The listing builds one solid part. Answer for the finished solid, in the listing's coordinates (mm). A direction names the side the tool comes from. Coordinates: 2 decimals unless noted, no trailing zeros. Order: outer loops, then holes, each group sorted by start corner. A loop starts at its lowest first (then second) coordinate and runs counter-clockwise, first axis right, second up. Notation, with made-up numbers: (71, 70.5) -> (102, 70.5) arc R15 ccw to (102, 76.5) -> close; hole circle Ø6 at (11.5, -6.75). An arc over 180 degrees is marked (long way). Answer in a Markdown table with one row per item.
```python
from build123d import *

# Parameters (mm, degrees)
SKETCH_1_W                = 5
SKETCH_1_H                = 10
EXTRUDE_1_DEPTH           = 4
CUT_EXTRUDE_1_DEPTH       = 9.124038405
CUT_EXTRUDE_1_DEPTH_BACK  = 9.124038405
CUT_EXTRUDE_2_DEPTH       = 9.124038405
CUT_EXTRUDE_2_DEPTH_BACK  = 9.124038405
SKETCH_6_W                = 4
SKETCH_6_H                = 3
CUT_EXTRUDE_3_DEPTH       = 2.5
SKETCH_7_W                = 4
SKETCH_7_H                = 3
CUT_EXTRUDE_4_DEPTH       = 2.5
CUT_EXTRUDE_5_DEPTH       = 9.124038405
CUT_EXTRUDE_5_DEPTH_BACK  = 9.124038405
CUT_EXTRUDE_10_DEPTH      = 9.124038405
CUT_EXTRUDE_10_DEPTH_BACK = 5
SKETCH_11_R               = 0.25
CUT_EXTRUDE_11_DEPTH      = 5
SKETCH_12_R               = 0.25
CUT_EXTRUDE_12_DEPTH      = 5
EXTRUDE_3_DEPTH           = 5
SCALE_1_SCALE             = 2.454545455


with BuildPart() as part:
    # Sketch 1 → Extrude 1 (new body)
    with BuildSketch(Plane.XY):
        Rectangle(SKETCH_1_W, SKETCH_1_H)
    extrude(amount=EXTRUDE_1_DEPTH)

    # Sketch 2 → Cut-Extrude 1 (cut, two sides: drawn at the far end of the back side and taken through both)
    with BuildSketch(Plane(origin=(2.5, 0, 0), x_dir=(0, 0, -1), z_dir=(1, 0, 0)).offset(-CUT_EXTRUDE_1_DEPTH_BACK)):
        Polygon((-31.620459958, -9.310229979), (-4, 4.5), (-3, 5), (24.620459958, 18.810229979), (-3, 74.051149895), (-59.240919916, 45.930689937), align=None)
    extrude(amount=CUT_EXTRUDE_1_DEPTH + CUT_EXTRUDE_1_DEPTH_BACK, mode=Mode.SUBTRACT)

    # Sketch 3 → Cut-Extrude 2 (cut, two sides: drawn at the far end of the back side and taken through both)
    with BuildSketch(Plane(origin=(2.5, 0, 0), x_dir=(0, 0, -1), z_dir=(1, 0, 0)).offset(-CUT_EXTRUDE_2_DEPTH_BACK)):
        Polygon((-3, 35.880613018), (-3, 5), (-3, -1), (0, -1), (30.880613018, -1), (76.363050598, 40.782734631), (42.48243758, 77.663347649), align=None)
    extrude(amount=CUT_EXTRUDE_2_DEPTH + CUT_EXTRUDE_2_DEPTH_BACK, mode=Mode.SUBTRACT)

    # Sketch 6 → Cut-Extrude 3 (cut)
    with BuildSketch(Plane(origin=(0, -1, 0), x_dir=(1, 0, 0), z_dir=(0, 1, 0))):
        with Locations((0, -1.5)):
            Rectangle(SKETCH_6_W, SKETCH_6_H)
    extrude(amount=-CUT_EXTRUDE_3_DEPTH, mode=Mode.SUBTRACT)

    # Sketch 7 → Cut-Extrude 4 (cut)
    with BuildSketch(Plane(origin=(0, 0, 3), x_dir=(-1, 0, 0), z_dir=(0, 0, -1))):
        with Locations((0, 3.5)):
            Rectangle(SKETCH_7_W, SKETCH_7_H)
    extrude(amount=-CUT_EXTRUDE_4_DEPTH, mode=Mode.SUBTRACT)

    # Sketch 8 → Cut-Extrude 5 (cut, two sides: drawn at the far end of the back side and taken through both)
    with BuildSketch(Plane(origin=(2.5, 0, 0), x_dir=(0, 0, -1), z_dir=(1, 0, 0)).offset(-CUT_EXTRUDE_5_DEPTH_BACK)):
        Polygon((-25.835890872, 17.835890872), (-4, -4), (-3, -5), (18.835890872, -26.835890872), (-24.835890872, -70.507672616), (-69.507672616, -25.835890872), align=None)
    extrude(amount=CUT_EXTRUDE_5_DEPTH + CUT_EXTRUDE_5_DEPTH_BACK, mode=Mode.SUBTRACT)

    # Sketch 9 → Cut-Extrude 10 (cut, two sides: drawn at the far end of the back side and taken through both)
    with BuildSketch(Plane(origin=(2.5, 0, 0), x_dir=(0, 0, -1), z_dir=(1, 0, 0)).offset(-CUT_EXTRUDE_10_DEPTH_BACK)):
        Polygon((-23.148447549, -26.648447549), (-1.5, -5), (0, -3.5), (21.648447549, 18.148447549), (64.945342647, -25.148447549), (20.148447549, -69.945342647), align=None)
    extrude(amount=CUT_EXTRUDE_10_DEPTH + CUT_EXTRUDE_10_DEPTH_BACK, mode=Mode.SUBTRACT)

    # Sketch 11 → Cut-Extrude 11 (cut)
    with BuildSketch(Plane(origin=(2.5, 0, 0), x_dir=(0, 0, -1), z_dir=(1, 0, 0))):
        with Locations(Location((-3.451895846, 3.5, 0), (0, 0, 90))):
            Circle(SKETCH_11_R)
    extrude(amount=-CUT_EXTRUDE_11_DEPTH, mode=Mode.SUBTRACT)

    # Sketch 12 → Cut-Extrude 12 (cut)
    with BuildSketch(Plane(origin=(2.5, 0, 0), x_dir=(0, 0, -1), z_dir=(1, 0, 0))):
        with Locations(Location((-0.5, -1.4, 0), (0, 0, 90))):
            Circle(SKETCH_12_R)
    extrude(amount=-CUT_EXTRUDE_12_DEPTH, mode=Mode.SUBTRACT)

    # Sketch 14 → Extrude 3 (add)
    with BuildSketch(Plane.ZY.offset(2.5)):
        Polygon((1.5, -5), (-1.5, -5), (-1.5, -3.5), (0, -3.5), align=None)
    extrude(amount=-EXTRUDE_3_DEPTH)


with BuildPart() as part_1:
    # Scale 1: scaled about (0, -2.526255673, 2.085256103)
    add(part.part.scale(SCALE_1_SCALE).moved(Location((0, 3.674553706, -3.033099786))))


solid = part_1.part
```
(1) A cutting plane is placed at B-B, the plane x = -3.5. Determine the outline of the cut face in (y, z).
Check values:
| item | result |
|---|---|
| outline | (-8.6, -6.71) -> (-4.92, -6.71) -> (-4.92, 4.33) -> (8.58, 4.33) -> (8.58, 6.79) -> (-6.14, 6.79) -> (-8.6, 4.33) -> close |
(2) A cutting plane is placed at C-C, the plane z = -1.5. Determine the outline of the cut face in (x, y).
Check values:
| item | result |
|---|---|
| outline | (-6.14, -8.6) -> (6.14, -8.6) -> (6.14, -0.29) -> (4.91, -0.29) -> (4.91, -4.92) -> (-4.91, -4.92) -> (-4.91, -0.29) -> (-6.14, -0.29) -> close; (-6.14, 0.77) -> (-4.91, 0.77) -> (-4.91, 1.22) -> (-6.14, 1.22) -> close; (4.91, 0.77) -> (6.14, 0.77) -> (6.14, 1.22) -> (4.91, 1.22) -> close |
(3) A cutting plane is placed at D-D, the plane z = 3. Determine the outline of the cut face in (x, y).
Check values:
| item | result |
|---|---|
| outline | (-6.14, -8.6) -> (6.14, -8.6) -> (6.14, 1.22) -> (4.91, 1.22) -> (4.91, -4.92) -> (-4.91, -4.92) -> (-4.91, 1.22) -> (-6.14, 1.22) -> close |
(4) For a pull along Z with two mould halves and no side action, classify faces 1 (the flat face through (0, -4.916, -1)), 2 (the cylindrical face through (-5.51, 12.83, 5.2)), 3 (the flat face through (-5.5, -1.8, -3.033)), 4 (the cylindrical face through (5.531, 0.105, -2.405)) as released by +Z, released by -Z, zero draft, split by the parting line, or undercut.
Check values:
| item | result |
|---|---|
| face 1 | zero draft |
| face 2 | undercut |
| face 3 | released by -Z |
| face 4 | undercut |
(5) Flat-ended cylindrical pins translate along their axes: pin 1 (0.6 mm diameter, centred on x = -5.5, y = -2, fed in from -Z); pin 2 (1.4 mm diameter, centred on x = 5.5, z = 2, fed in from +Y); pin 3 (3.5 mm diameter, centred on x = -2, z = 0.5, fed in from +Y); pin 4 (1.4 mm diameter, centred on y = 12.27, z = 5.44, fed in from -X). Find the tip coordinate at first contact, or state that the pin passes through.
Check values:
| item | result |
|---|---|
| pin 1 | z = -3.03 |
| pin 2 | y = 1.22 |
| pin 3 | y = -4.92 |
| pin 4 | x = -6.14 |
(6) A cutting plane is placed at A-A, the plane y = 13.25. Determine the outline of the cut face in (x, z), then the cut area to 3 significant figures.
Check values:
| item | result |
|---|---|
| outline | (-6.14, 4.33) -> (-4.91, 4.33) -> (-4.91, 6.79) -> (-6.14, 6.79) -> close; (4.91, 4.33) -> (6.14, 4.33) -> (6.14, 6.79) -> (4.91, 6.79) -> close |
| area | 6.02 mm² |
(7) Find the intervals of material crossed by line 1 along Z through (x, y) = (-4, -4.5); line 2 along Y through (x, z) = (-2.5, 0.25); line 3 along Y through (x, z) = (-5, 4), in increasing order. Write a range as from..to.
Check values:
| item | result |
|---|---|
| line 1 | 4.33..6.79 |
| line 2 | -8.6..-4.92 |
| line 3 | -8.6..1.22 |
(8) Which of the six approach directions +Z, -Z, +X, -X, +Y, -Y give full straight-line access (tool end or side, diameter ignored) to faces 5 (the flat face through (5.5, 1.22, 0.7)), 6 (the flat face through (-4.909, -2, 1)), 7 (the flat face through (4.909, 11, 6)), 8 (the flat face through (0, -7, -6.715))?
Check values:
| item | result |
|---|---|
| face 5 | -Z, +X, -X, +Y |
| face 6 | -Z, +Y |
| face 7 | +Z, -Z, +Y |
| face 8 | -Z, +X, -X, +Y, -Y |
